The model under review builds one solid part; all positions refer to its coordinate system, in mm. Face numbers are marked on the shaded views. A direction names the side the tool comes from. Coordinates: 2 decimals unless noted, no trailing zeros. Write each loop counter-clockwise with the first axis right and the second up, starting at its lowest first coordinate (ties: lowest second). Pieces come first, ordered by that corner, then holes.
1) Add section C-C, the plane y = 0.75. State the section outline as (x, z) points.
2) Add section B-B, the plane x = 0. State the section outline as (y, z) points, then the cut area to 3 significant figures.
3) Mouldability with a two-part tool opening along X and no side actions: class the marked faces 6, 7, 8 and 9 as released by +X, released by -X, zero draft, split by the parting line, or undercut.
4) For P1, Ø0.9, axis at x = -10.5, y = 2, coming from the +Z side; P2, Ø1.5, axis at x = -12.5, y = 2, coming from the -Z side, all flat-tipped, find the tip position at first contact; note any pin that passes through.
5) Machinability: for the marked faces 1, 2, 3, 4 and 5, which of the approach directions +Z, -Z, +X, -X, +Y, -Y give a long, thin tool a straight path to every point of the face, cutting with its end or side? Answer none if there is none.
6) For line 1 (X direction, y = 1.5, z = 0); line 2 (Z direction, x = 8, y = 0.85); line 3 (Z direction, x = -2.5, y = 2.6), list the stretches that pass through material, from the lowest coordinate up.
7) Add section A-A, the plane z = 0. State the section outline as (x, y) points, then the cut area to 3 significant figures.
8) Add section D-D, the plane x = 12. State the section outline as (y, z) points.
from build123d import *

# Parameters (mm, degrees)
SKETCH1_R           = 7.25
SKETCH1_R_2         = 4.35
BOSS_EXTRUDE1_DEPTH = 3
SKETCH2_W           = 14
SKETCH2_H           = 6
BOSS_EXTRUDE2_DEPTH = 3


with BuildPart() as part:
    # Sketch1 → Boss-Extrude1 (new body)
    with BuildSketch(Plane(origin=(0, 0, 0), x_dir=(1, 0, 0), z_dir=(0, 1, 0))):
        with Locations(Location((0, 0, 0), (0, 0, 270))):
            Circle(SKETCH1_R)
        with Locations(Location((0, 0, 0), (0, 0, 270))):
            Circle(SKETCH1_R_2, mode=Mode.SUBTRACT)
    extrude(amount=BOSS_EXTRUDE1_DEPTH)

    # Sketch2 → Boss-Extrude2 (add)
    with BuildSketch(Plane(origin=(0, 0, 0), x_dir=(1, 0, 0), z_dir=(0, 1, 0))):
        Polygon((4.35, 3), (4.35, 0), (4.35, -3), (18.35, -3), (18.35, 3), align=None)
        with Locations((-11.35, 0)):
            Rectangle(SKETCH2_W, SKETCH2_H)
    extrude(amount=BOSS_EXTRUDE2_DEPTH)


solid = part.part
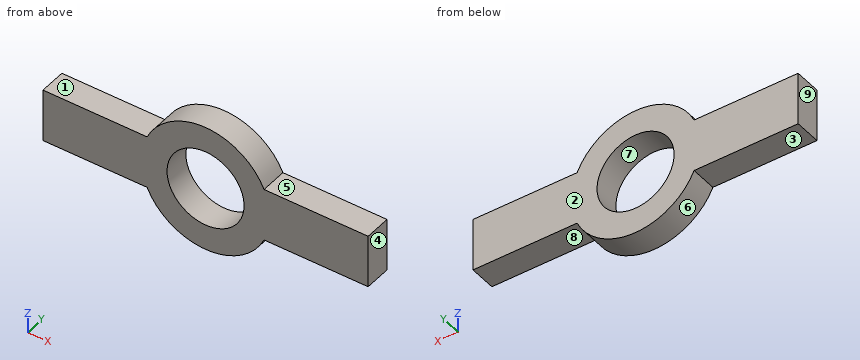
Geometry results:
1. outline: (-18.35, -3) - (-6.6, -3) arc R7.25 ccw to (6.6, -3) - (18.35, -3) - (18.35, 3) - (6.6, 3) arc R7.25 ccw to (-6.6, 3) - (-18.35, 3) - close; hole circle Ø8.7 at (0, 0)
2. outline: (0, -7.25) - (3, -7.25) - (3, -4.35) - (0, -4.35) - close; (0, 4.35) - (3, 4.35) - (3, 7.25) - (0, 7.25) - close
2. area: 17.4 mm2
3. face 6: split by the parting line
3. face 7: undercut
3. face 8: zero draft
3. face 9: released by -X
4. P1: stops at z = 3
4. P2: stops at z = -3
5. face 1: +Z, -X, +Y, -Y
5. face 2: +Z, -Z, +X, -X, +Y
5. face 3: -Z, -X, +Y, -Y
5. face 4: +Z, -Z, +X, +Y, -Y
5. face 5: +Z, +X, +Y, -Y
6. line 1: x = -18.35 to -4.35, 4.35 to 18.35
6. line 2: z = -3 to 3
6. line 3: z = -6.81 to -3.56, 3.56 to 6.81
7. outline: (-18.35, 0) - (-4.35, 0) - (-4.35, 3) - (-18.35, 3) - close; (4.35, 0) - (18.35, 0) - (18.35, 3) - (4.35, 3) - close
7. area: 84.0 mm2
8. outline: (0, -3) - (3, -3) - (3, 3) - (0, 3) - close
